The listing builds one solid part. Answer for the finished solid, in the listing's coordinates (mm). A direction names the side the tool comes from. Round coordinates to 2 decimals unless told otherwise and drop trailing zeros. Write each loop counter-clockwise with the first axis right and the second up, starting at its lowest first coordinate (ties: lowest second). Pieces come first, ordered by that corner, then holes. Notation, with made-up numbers: M 10,45 L 48,45 A13 cw 48,66 Z; hole C 55,62 d6. An arc over 180 degrees is marked long. Answer as CSV lines item,"result". Start each with the question number.
from build123d import *

# Parameters (mm, degrees)
CROQUIS1_W              = 3
CROQUIS1_H              = 7.7
CROQUIS1_W_2            = 7.7
CROQUIS1_H_2            = 3
CROQUIS1_W_3            = 40
CROQUIS1_H_3            = 40
SALIENTE_EXTRUIR1_DEPTH = 3


with BuildPart() as part:
    # Croquis1 → Saliente-Extruir1 (new body)
    with BuildSketch(Plane.XY):
        with Locations((-21.5, -7.95)):
            Rectangle(CROQUIS1_W, CROQUIS1_H)
        with Locations((-7.95, -21.5)):
            Rectangle(CROQUIS1_W_2, CROQUIS1_H_2)
        with Locations((7.95, -21.5)):
            Rectangle(CROQUIS1_W_2, CROQUIS1_H_2)
        with Locations((21.5, -7.95)):
            Rectangle(CROQUIS1_W, CROQUIS1_H)
        with Locations((21.5, 7.95)):
            Rectangle(CROQUIS1_W, CROQUIS1_H)
        with Locations((-21.5, 7.95)):
            Rectangle(CROQUIS1_W, CROQUIS1_H)
        with Locations((-7.95, 21.5)):
            Rectangle(CROQUIS1_W_2, CROQUIS1_H_2)
        with Locations((7.95, 21.5)):
            Rectangle(CROQUIS1_W_2, CROQUIS1_H_2)
        Rectangle(CROQUIS1_W_3, CROQUIS1_H_3)
    extrude(amount=SALIENTE_EXTRUIR1_DEPTH)


solid = part.part
Q1. The mould has two halves that part along X. Classify faces 1 (the face through (4.1, 21, 1)), 2 (the face through (-23, 8, 1)), 3 (the face through (-8, 23, 1)), 4 (the face through (0, -20, 1)): +X half, -X half, draft (parallel to the pull), parting line (faces both ways), or undercut.
Q2. Each of these flat-tipped pins is pushed along its axis until it touches: P1, Ø0.9, axis at y = -17.5, z = 2, coming from the -X side; P2, Ø1.5, axis at x = -17, z = 2, coming from the +Y side; P3, Ø4, axis at x = -0.5, y = 4.5, coming from the -Z side; P4, Ø1.5, axis at x = 17.5, z = 1.5, coming from the -Y side. Where does it stop, or does it pass through?
Q3. For faces 5 (the face through (0, 20, 1)), 6 (the face through (21, 4.1, 1)), 7 (the face through (20, -16, 1)), determine the directions among +Z, -Z, +X, -X, +Y, -Y from which every point of the face is accessible in a straight line to the end or side of a thin tool.
Q4. Find section A-A (x = 19). Determine the outline of the cut face in (y, z), plus the area to 3 significant figures.
Q5. Straight lines are drawn through the part: L1, parallel to Y at x = 12, z = 1.5; L2, parallel to Y at x = 21, z = 1.9. For each, find the intervals that lie inside material, in ascending order.
Reported:
1,face 1,"undercut"
1,face 2,"-X half"
1,face 3,"draft"
1,face 4,"undercut"
2,P1,"stops at x = -20"
2,P2,"stops at y = 20"
2,P3,"stops at z = 0"
2,P4,"stops at y = -20"
3,face 5,"+Z, -Z, +Y"
3,face 6,"+Z, -Z, +X"
3,face 7,"+Z, -Z, +X, -Y"
4,outline,"M -20,0 L 20,0 L 20,3 L -20,3 Z"
4,area,"120 mm2"
5,L1,"y = -20 to 20"
5,L2,"y = -11.8 to -4.1, 4.1 to 11.8"
